Design review of the part built by this model. Coordinates are the model's own, in mm. Face numbers are marked on the shaded views. A direction names the side the tool comes from. Coordinates: 2 decimals unless noted, no trailing zeros. Order: outer loops, then holes, each group sorted by start corner. A loop starts at its lowest first (then second) coordinate and runs counter-clockwise, first axis right, second up. Notation, with made-up numbers: (3, 9) -> (28, 9) arc R32 cw to (28, 38) -> close; hole circle Ø5 at (61, 28.5). An arc over 180 degrees is marked (long way). Use a Markdown table: item, result. Add a question column.
Q1. Wall thickness on probe 1 along Z at (x, y) = (0, 4.75); probe 2 along X at (y, z) = (-7, 0.25); probe 3 along Z at (x, y) = (3.5, -41): over which ranges is each line inside the solid? List them lowest first.
Q2. Add section B-B (x = 0). State the section outline as (y, z) points.
Q3. Add section A-A (z = 0). State the section outline as (x, y) points.
Q4. Add section D-D (y = -45.75). State the section outline as (x, z) points, then the cut area to 3 significant figures.
Q5. Machinability: for the marked faces 1 and 2, which of the approach directions +Z, -Z, +X, -X, +Y, -Y give a long, thin tool a straight path to every point of the face, cutting with its end or side? Answer none if there is none.
Q6. Add section C-C (y = 4). State the section outline as (x, z) points, then the cut area to 3 significant figures.
Q7. Insertion check: pin 1 (1.5 mm diameter, centred on y = -18, z = -1.5, fed in from -X); pin 2 (3 mm diameter, centred on x = -3, y = -31, fed in from -Z); pin 3 (4 mm diameter, centred on x = 3.5, y = -20.5, fed in from +Z); pin 4 (5 mm diameter, centred on x = 0, z = 0, fed in from -Y). Each pin has a flat end and moves straight along its axis. Give the tip position at first contact, or say it passes through.
from build123d import *

# Parameters (mm, degrees)
F3_R      = 4.7
F4_DEPTH  = 42
F8_DEPTH  = 42
F6_R      = 4.7
F6_R_2    = 4
F9_DEPTH  = 10
F7_R      = 4.7
F7_R_2    = 4
F10_DEPTH = 12
F11_R     = 2.75
F12_DEPTH = 4.701


# Not quite as in the source:
# - ends of sketch curves that miss each other by under 0.0002 mm in the source are joined


with BuildPart() as f4:
    # F3 (on Front) → F4 (new body)
    with BuildSketch(Plane.XZ):
        Circle(F3_R)
    extrude(amount=F4_DEPTH)

    # F5 (on face) → F8 (cut, through all)
    with BuildSketch(Plane.XZ.offset(42)):
        with BuildLine():
            Line((-1.25, -3.8), (0, -3.8))
            Line((0, -3.8), (1.25, -3.8))
            Line((1.25, -3.8), (1.25, -3.7))
            ThreePointArc((1.25, -3.7), (1.3085786438, -3.5585786438), (1.45, -3.5))
            Line((1.45, -3.5), (2, -3.5))
            Line((2, -3.5), (2, -3.05))
            ThreePointArc((2, -3.05), (2.0585786438, -2.9085786438), (2.2, -2.85))
            Line((2.2, -2.85), (3.15, -2.85))
            Line((3.15, -2.85), (3.15, -2.15))
            Line((3.15, -2.15), (2.2, -2.15))
            ThreePointArc((2.2, -2.15), (2.0585786438, -2.0914213562), (2, -1.95))
            Line((2, -1.95), (2, -1.887459))
            ThreePointArc((2, -1.887459), (2.1033535752, -1.771554046), (2.2, -1.65))
            Line((2.2, -1.65), (3.75, -1.65))
            Line((3.75, -1.65), (3.75, 0))
            Line((3.75, 0), (3.75, 1.65))
            Line((3.75, 1.65), (2.2, 1.65))
            ThreePointArc((2.2, 1.65), (2.1033535752, 1.771554046), (1.9999998047, 1.8874588157))
            Line((1.9999998047, 1.8874588157), (2, 1.95))
            ThreePointArc((2, 1.95), (2.0585786438, 2.0914213562), (2.2, 2.15))
            Line((2.2, 2.15), (3.15, 2.15))
            Line((3.15, 2.15), (3.15, 2.85))
            Line((3.15, 2.85), (2.2, 2.85))
            ThreePointArc((2.2, 2.85), (2.0585786438, 2.9085786438), (2, 3.05))
            Line((2, 3.05), (2, 3.5))
            Line((2, 3.5), (1.45, 3.5))
            ThreePointArc((1.45, 3.5), (1.3085786438, 3.5585786438), (1.25, 3.7))
            Line((1.25, 3.7), (1.25, 3.8))
            Line((1.25, 3.8), (0, 3.8))
            Line((0, 3.8), (-1.25, 3.8))
            Line((-1.25, 3.8), (-1.25, 3.7))
            ThreePointArc((-1.25, 3.7), (-1.3085786438, 3.5585786438), (-1.45, 3.5))
            Line((-1.45, 3.5), (-2, 3.5))
            Line((-2, 3.5), (-2, 3.05))
            ThreePointArc((-2, 3.05), (-2.0585786438, 2.9085786438), (-2.2, 2.85))
            Line((-2.2, 2.85), (-3.15, 2.85))
            Line((-3.15, 2.85), (-3.15, 2.15))
            Line((-3.15, 2.15), (-2.2, 2.15))
            ThreePointArc((-2.2, 2.15), (-2.0585786438, 2.0914213562), (-2, 1.95))
            Line((-2, 1.95), (-2, 1.887459))
            ThreePointArc((-2, 1.887459), (-2.1033535752, 1.771554046), (-2.2, 1.65))
            Line((-2.2, 1.65), (-3.75, 1.65))
            Line((-3.75, 1.65), (-3.75, 0))
            Line((-3.75, 0), (-3.75, -1.65))
            Line((-3.75, -1.65), (-2.2, -1.65))
            ThreePointArc((-2.2, -1.65), (-2.1033535752, -1.771554046), (-1.9999998047, -1.8874588157))
            Line((-1.9999998047, -1.8874588157), (-2, -1.95))
            ThreePointArc((-2, -1.95), (-2.0585786438, -2.0914213562), (-2.2, -2.15))
            Line((-2.2, -2.15), (-3.15, -2.15))
            Line((-3.15, -2.15), (-3.15, -2.85))
            Line((-3.15, -2.85), (-2.2, -2.85))
            ThreePointArc((-2.2, -2.85), (-2.0585786438, -2.9085786438), (-2, -3.05))
            Line((-2, -3.05), (-2, -3.5))
            Line((-2, -3.5), (-1.45, -3.5))
            ThreePointArc((-1.45, -3.5), (-1.3085786438, -3.5585786438), (-1.25, -3.7))
            Line((-1.25, -3.7), (-1.25, -3.8))
        make_face()
    extrude(amount=-F8_DEPTH, mode=Mode.SUBTRACT)

    # F6 (on face) → F9 (join)
    with BuildSketch(Plane.XZ.offset(42)):
        Circle(F6_R)
        Circle(F6_R_2, mode=Mode.SUBTRACT)
    extrude(amount=F9_DEPTH)

    # F7 (on face) → F10 (join)
    with BuildSketch(Plane(origin=(0, 0, 0), x_dir=(-1, 0, 0), z_dir=(0, 1, 0))):
        Circle(F7_R)
        Circle(F7_R_2, mode=Mode.SUBTRACT)
    extrude(amount=F10_DEPTH)

    # F11 (on Right) → F12 (cut, through all)
    with BuildSketch(Plane.YZ):
        with Locations((-45.75, 0)):
            Circle(F11_R)
    extrude(amount=-F12_DEPTH, mode=Mode.SUBTRACT)


solid = f4.part
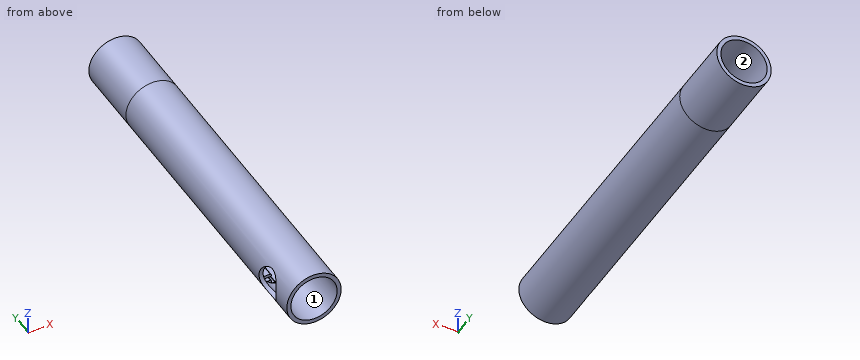
Established:
| question | item | result |
|---|---|---|
| 1 | probe 1 | -4.7 to -4, 4 to 4.7 |
| 1 | probe 2 | -4.69 to -3.75, 3.75 to 4.69 |
| 1 | probe 3 | -3.14 to -1.65, 1.65 to 3.14 |
| 2 | outline | (-52, -4.7) -> (12, -4.7) -> (12, -4) -> (0, -4) -> (0, -3.8) -> (-42, -3.8) -> (-42, -4) -> (-52, -4) -> close; (-52, 4) -> (-42, 4) -> (-42, 3.8) -> (0, 3.8) -> (0, 4) -> (12, 4) -> (12, 4.7) -> (-52, 4.7) -> close |
| 3 | outline | (-4.7, -52) -> (-4, -52) -> (-4, -48.5) -> (-4.7, -48.5) -> close; (-4.7, -43) -> (-4, -43) -> (-4, -42) -> (-3.75, -42) -> (-3.75, 0) -> (-4, 0) -> (-4, 12) -> (-4.7, 12) -> close; (3.75, -42) -> (4, -42) -> (4, -52) -> (4.7, -52) -> (4.7, 12) -> (4, 12) -> (4, 0) -> (3.75, 0) -> close |
| 4 | outline | (-3.81, -2.75) arc R4.7 ccw (long way) to (-3.81, 2.75) -> (-2.9, 2.75) arc R4 cw (long way) to (-2.9, -2.75) -> close |
| 4 | area | 15.0 mm^2 |
| 5 | face 1 | -Y |
| 5 | face 2 | +Y |
| 6 | outline | circle Ø9.4 at (0, 0); hole circle Ø8 at (0, 0) |
| 6 | area | 19.1 mm^2 |
| 7 | pin 1 | x = -4.64 |
| 7 | pin 2 | z = -4.45 |
| 7 | pin 3 | z = 4.45 |
| 7 | pin 4 | through |
